from build123d import *

# Parameters (mm, degrees)
SKETCH_1_W          = 25
SKETCH_1_H          = 41
EXTRUDE_1_DEPTH     = 42.5
FILLET_1_R          = 1
SKETCH_2_R          = 24.95
CUT_EXTRUDE_1_DEPTH = 42.5
SKETCH_3_R          = 2.5
CUT_EXTRUDE_2_DEPTH = 10


with BuildPart() as part:
    # Эскиз1 → Бобышка-Вытянуть1 (new body)
    with BuildSketch(Plane(origin=(0, 0, 0), x_dir=(1, 0, 0), z_dir=(0, 1, 0))):
        Rectangle(SKETCH_1_W, SKETCH_1_H)
    extrude(amount=EXTRUDE_1_DEPTH)

    # Скругление1
    fillet_1_edges = [part.edges().sort_by_distance(p)[0] for p in [
        (-12.5, 0, 0),
    ]]
    fillet(fillet_1_edges, radius=FILLET_1_R)

    # Эскиз2 → Вырез-Вытянуть1 (cut)
    with BuildSketch(Plane(origin=(0, 42.5, 0), x_dir=(1, 0, 0), z_dir=(0, 1, 0))):
        with Locations((12.5, 0)):
            Circle(SKETCH_2_R)
    extrude(amount=-CUT_EXTRUDE_1_DEPTH, mode=Mode.SUBTRACT)

    # Эскиз3 → Вырез-Вытянуть2 (cut)
    with BuildSketch(Plane.ZY.offset(12.5)):
        with Locations((-12.5, 25)):
            Circle(SKETCH_3_R)
        with Locations((0, 37.5)):
            Circle(SKETCH_3_R)
        with Locations((12.5, 25)):
            Circle(SKETCH_3_R)
        with Locations((0, 12.5)):
            Circle(SKETCH_3_R)
        with Locations((0, 25)):
            Circle(SKETCH_3_R)
    extrude(amount=-CUT_EXTRUDE_2_DEPTH, mode=Mode.SUBTRACT)


solid = part.part
Could you check a few things on this model? Use its own coordinates, in mm. Give positions to 0.01 mm unless a question says otherwise; leave off trailing zeros. Order: outer loops, then holes, each group sorted by start corner. A loop starts at its lowest first (then second) coordinate and runs counter-clockwise, first axis right, second up.
1. Will these pins go through, and if not, where does the flat tip stop? P1, Ø6, axis at y = 25, z = 12.5, coming from the +X side; P2, Ø3, axis at y = 12.5, z = 0, coming from the +X side; P3, Ø4, axis at y = 34.5, z = -4.5, coming from the +X side; P4, Ø8, axis at y = 31.5, z = 0, coming from the +X side.
2. Suppose I cut it at A-A (y = 37.5). List the corners of the cut face in (x, z) for me, plus the area to 3 significant figures.
3. We'd pull the mould along Z, two halves only. Please class faces 1 (the cylindrical face through (-11.949, 21.548, 4.976)), 2 (the flat face through (-12.5, 21, 5)), 3 (the flat face through (-7, 21, 20.5)): pulls with the +Z half, pulls with the -Z half, needs draft (parallel to the pull), parting line crosses it, or undercut.
4. I need wall thicknesses on L1, parallel to Z at x = -12.4, y = 25; L2, parallel to Y at x = -9.5, z = 12.5; L3, parallel to Z at x = -9, y = 25. Which ranges of each line are inside material? Lowest first, please.
5. Suppose I cut it at C-C (z = -12.5). List the corners of the cut face in (x, y) for me.
6. Suppose I cut it at D-D (x = -11). List the corners of the cut face in (y, z) for me, plus the area to 3 significant figures.
7. Suppose I cut it at B-B (x = -4). List the corners of the cut face in (y, z) for me.
Solved:
1. P1: stops at x = -7.05
1. P2: passes through
1. P3: stops at x = -11.59
1. P4: stops at x = -12.13
2. outline: (-12.5, -20.5) - (-1.72, -20.5) arc R24.95 cw to (-12.32, -2.5) - (-12.5, -2.5) - close; (-12.5, 2.5) - (-12.32, 2.5) arc R24.95 cw to (-1.72, 20.5) - (-12.5, 20.5) - close
2. area: 133 mm2
3. face 1: undercut
3. face 2: needs draft
3. face 3: pulls with the +Z half
4. L1: z = -20.5 to -15, -10 to -2.5, 2.5 to 10, 15 to 20.5
4. L2: y = 0 to 22.5, 27.5 to 42.5
4. L3: z = -20.5 to -15, 15 to 20.5
5. outline: (-12.5, 1) arc R1 ccw to (-11.5, 0) - (-9.09, 0) - (-9.09, 22.5) - (-12.5, 22.5) - close; (-12.5, 27.5) - (-9.09, 27.5) - (-9.09, 42.5) - (-12.5, 42.5) - close
6. outline: (0, -20.5) - (42.5, -20.5) - (42.5, -8.38) - (0, -8.38) - close; (0, 8.38) - (42.5, 8.38) - (42.5, 20.5) - (0, 20.5) - close; hole circle Ø5 at (25, -12.5); hole circle Ø5 at (25, 12.5)
6. area: 991 mm2
7. outline: (0, -20.5) - (42.5, -20.5) - (42.5, -18.72) - (0, -18.72) - close; (0, 18.72) - (42.5, 18.72) - (42.5, 20.5) - (0, 20.5) - close
